Can you work these out from the drawing? Everything is in mm from the part's minimum corner. Round coordinates to 2 decimals unless told otherwise and drop trailing zeros. Write each loop counter-clockwise with the first axis right and the second up, starting at its lowest first coordinate (ties: lowest second). Pieces come first, ordered by that corner, then holes. Notation, with made-up numbers: (47.5, 81) -> (75.5, 81) arc R13 ccw to (75.5, 97) -> close; hole circle Ø10 at (52.25, 84.5). An arc over 180 degrees is marked (long way). Answer as CSV lines item,"result".
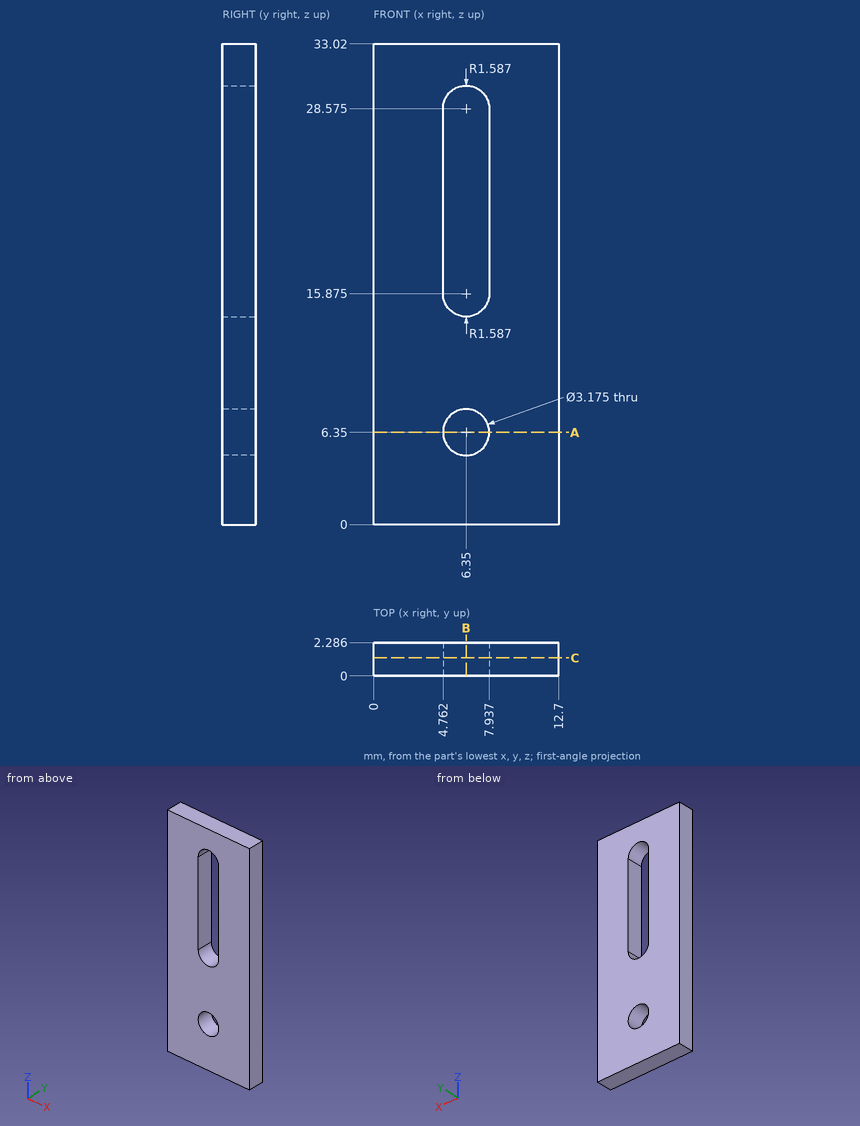
Item 1: I need wall thicknesses on L1, parallel to Z at x = 6.35, y = 0.7; L2, parallel to X at y = 1.3, z = 6.35; L3, parallel to Z at x = 5.25, y = 1.35 (1 decimal). Which ranges of each line are inside material? Lowest first, please.
Results found:
L1,"z = 0 to 4.76, 7.94 to 14.29, 30.16 to 33.02"
L2,"x = 0 to 4.76, 7.94 to 12.7"
L3,"z = 0 to 5.2, 7.5 to 14.7, 29.7 to 33"
Item 2: Suppose I cut it at A-A, the plane z = 6.35. List the corners of the cut face in (x, y) for me (1 decimal).
Results found:
outline,"(0, 0) -> (4.8, 0) -> (4.8, 2.3) -> (0, 2.3) -> close; (7.9, 0) -> (12.7, 0) -> (12.7, 2.3) -> (7.9, 2.3) -> close"
Item 3: Suppose I cut it at B-B, the plane x = 6.35. List the corners of the cut face in (y, z) for me (1 decimal).
Results found:
outline,"(0, 0) -> (2.3, 0) -> (2.3, 4.8) -> (0, 4.8) -> close; (0, 7.9) -> (2.3, 7.9) -> (2.3, 14.3) -> (0, 14.3) -> close; (0, 30.2) -> (2.3, 30.2) -> (2.3, 33) -> (0, 33) -> close"
Item 4: Will this pin go through, and if not, where does the flat tip stop? pin 1 (3 mm diameter, centred on x = 6.35, z = 6.35, fed in from -Y).
Results found:
pin 1,"passes through"
Item 5: Suppose I cut it at C-C, the plane y = 1.25. State how many separate pieces and enclosed holes the cut face has, then the cut area to 3 significant figures.
Results found:
separate pieces,"1"
enclosed holes,"2"
area,"363 mm²"
